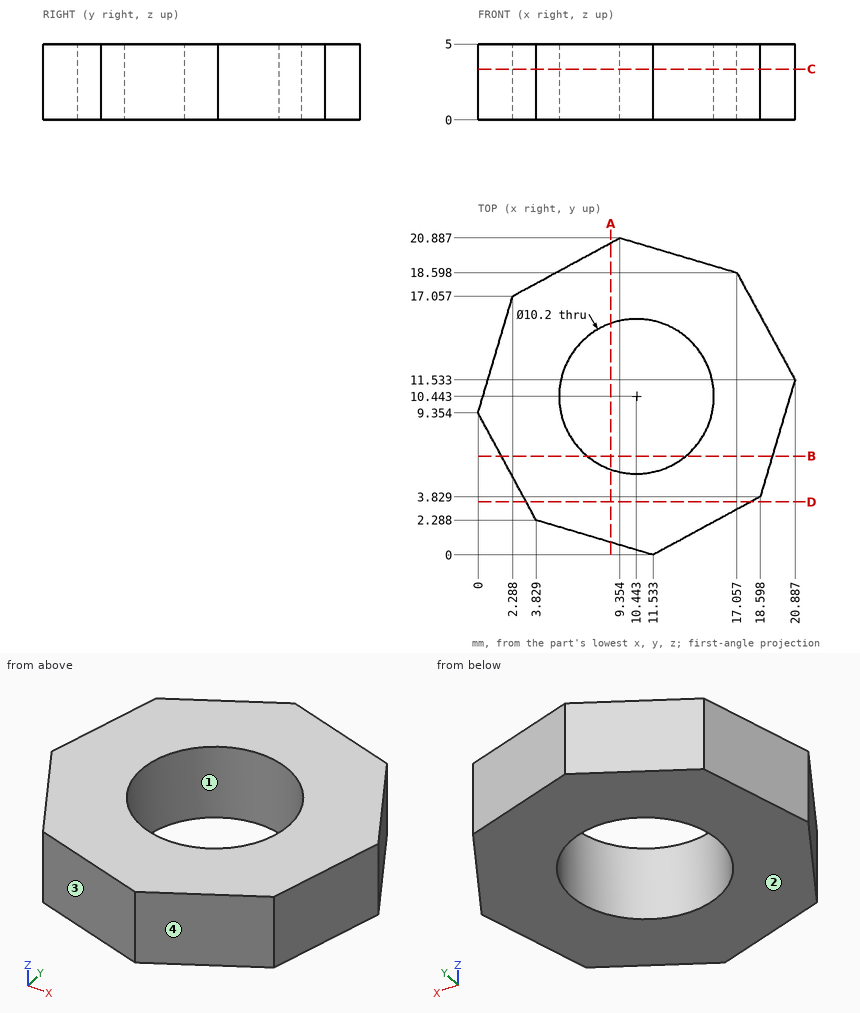
Can you work these out from the drawing? Everything is in mm from the part's minimum corner. Coordinates: 2 decimals unless noted, no trailing zeros. Loops run counter-clockwise (first coordinate to the right, second up) from the corner with the lowest first, then second, coordinate; pieces in that order, holes last. Notation, with made-up numbers: (-17.5, 86.5) - (32.5, 86.5) arc R15 cw to (32.5, 113.5) - close; hole circle Ø5 at (80, 74.5). An arc over 180 degrees is marked (long way). Answer as CSV lines item,"result".
Q1. For pin 1 (1.5 mm diameter, centred on y = 13, z = 3, fed in from -X); pin 2 (6 mm diameter, centred on x = 10, y = 8, fed in from +Z); pin 3 (6 mm diameter, centred on x = 10.44, y = 10.44, fed in from +Z), each with a flat end and sliding along its axis, tell me the tip position at first contact or that it passes through.
Response:
pin 1,"x = 0.86"
pin 2,"z = 5"
pin 3,"through"
Q2. If I drill on L1, parallel to Y at x = 12.5, z = 3.95 (1 decimal); L2, parallel to X at y = 12.5, z = 3.15 (1 decimal); L3, parallel to Y at x = 13.75, z = 4.4 (1 decimal), over which ranges is the centre line in solid material (lowest first)? Write a range as [from, to].
Response:
L1,"[0.5, 5.8], [15.1, 20]"
L2,"[0.9, 5.8], [15.1, 20.4]"
L3,"[1.2, 6.6], [14.3, 19.6]"
Q3. If we section it at A-A, the plane x = 8.75: Write out the boundary of the cut face in (y, z).
Response:
outline,"(0.83, 0) - (5.63, 0) - (5.63, 5) - (0.83, 5) - close; (15.25, 0) - (20.56, 0) - (20.56, 5) - (15.25, 5) - close"
Q4. If we section it at C-C, the plane z = 3.35: Write out the boundary of the cut face in (x, y), and give its area (3 significant figures).
Response:
outline,"(0, 9.35) - (3.83, 2.29) - (11.53, 0) - (18.6, 3.83) - (20.89, 11.53) - (17.06, 18.6) - (9.35, 20.89) - (2.29, 17.06) - close; hole circle Ø10.2 at (10.44, 10.44)"
area,"230 mm2"
Q5. If we section it at D-D, the plane y = 3.5: Write out the boundary of the cut face in (x, z), and give its area (3 significant figures).
Response:
outline,"(3.17, 0) - (17.99, 0) - (17.99, 5) - (3.17, 5) - close"
area,"74.1 mm2"
Q6. If we section it at B-B, the plane y = 6.5: Write out the boundary of the cut face in (x, z).
Response:
outline,"(1.55, 0) - (7.21, 0) - (7.21, 5) - (1.55, 5) - close; (13.68, 0) - (19.39, 0) - (19.39, 5) - (13.68, 5) - close"
Q7. We'd pull the mould along X, two halves only. Please class the marked faces 1, 2, 3 and 4: pulls with the +X half, pulls with the -X half, needs draft (parallel to the pull), parting line crosses it, or undercut.
Response:
face 1,"undercut"
face 2,"needs draft"
face 3,"pulls with the -X half"
face 4,"pulls with the +X half"
